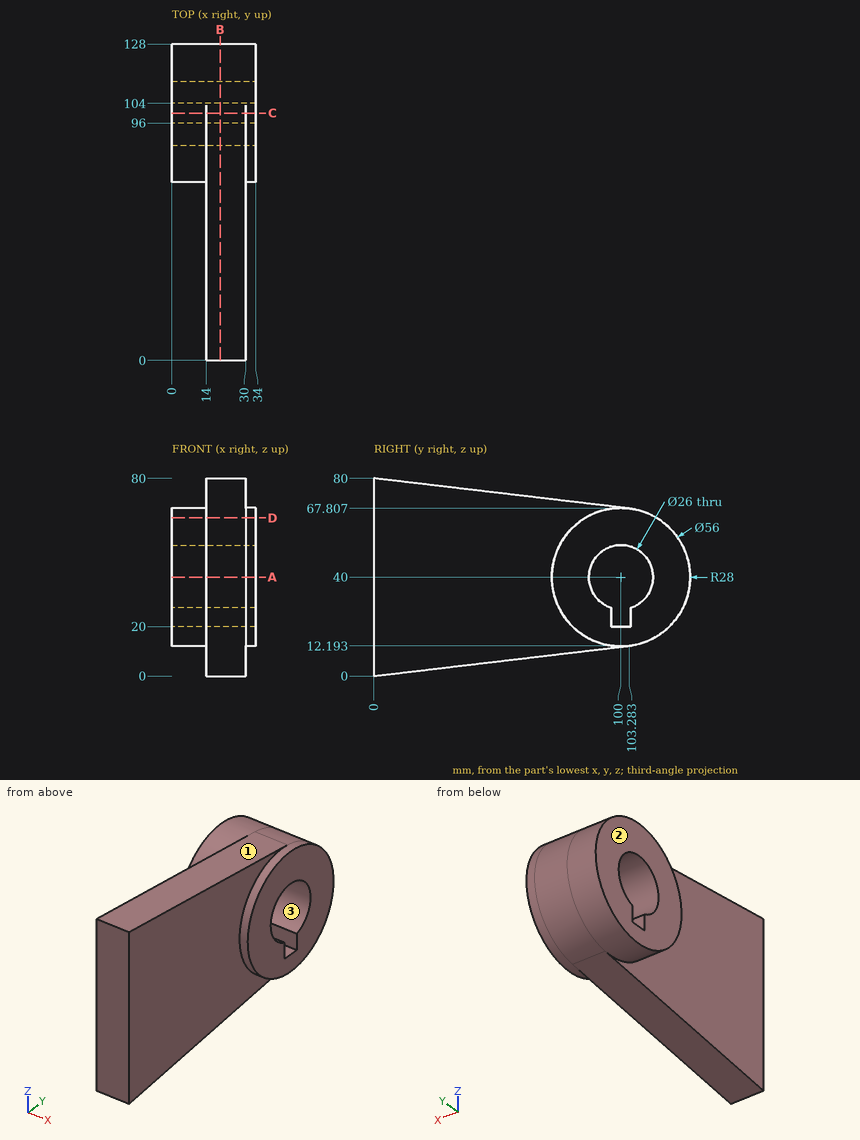
Print and shaded views of the part. All mm, measured from the part's lowest x, y and z. Coordinates: 2 decimals unless noted, no trailing zeros. Write each loop counter-clockwise with the first axis right and the second up, starting at its lowest first coordinate (ties: lowest second). Pieces come first, ordered by that corner, then holes.
(1) Two-plate mould, pull along Y, no slides. Class the marked faces 1, 2 and 3: +Y half, -Y half, draft (parallel to the pull), parting line (faces both ways), or undercut.
(2) Cut at A-A, the plane z = 40. List the corners of the cut face in (x, y).
(3) Cut at D-D, the plane z = 64. List the corners of the cut face in (x, y).
(4) Cut at C-C, the plane y = 100. List the corners of the cut face in (x, z).
(5) Flat gauge pins, fed straight in: pin 1 (2 mm diameter, centred on x = 25.5, y = 85.5, fed in from +Z); pin 2 (4 mm diameter, centred on x = 25.5, y = 52.5, fed in from +Z); pin 3 (5 mm diameter, centred on x = 5, z = 8, fed in from +Y); pin 4 (12 mm diameter, centred on x = 7.5, y = 109, fed in from -Z). Where does each tip first touch, or does it go through?
(6) Drill centre lines: probe 1 along Z at (x, y) = (11, 100); probe 2 along Y at (x, z) = (20, 40); probe 3 along Y at (x, z) = (13, 22). Where is each one in solid material? Low to high.
(7) Cut at B-B, the plane x = 19.5. List the corners of the cut face in (y, z).
Geometry says:
1. face 1: +Y half
1. face 2: draft
1. face 3: undercut
2. outline: (0, 72) - (14, 72) - (14, 0) - (30, 0) - (30, 72) - (34, 72) - (34, 87) - (0, 87) - close; (0, 113) - (34, 113) - (34, 128) - (0, 128) - close
3. outline: (0, 85.58) - (14, 85.58) - (14, 0) - (30, 0) - (30, 85.58) - (34, 85.58) - (34, 114.42) - (0, 114.42) - close
4. outline: (0, 12) - (14, 12) - (14, 11.81) - (30, 11.81) - (30, 12) - (34, 12) - (34, 20) - (0, 20) - close; (0, 53) - (34, 53) - (34, 68) - (30, 68) - (30, 68.19) - (14, 68.19) - (14, 68) - (0, 68) - close
5. pin 1: stops at z = 70.02
5. pin 2: stops at z = 74.04
5. pin 3: passes through
5. pin 4: stops at z = 12.16
6. probe 1: z = 12 to 20, 53 to 68
6. probe 2: y = 0 to 87, 113 to 128
6. probe 3: y = 78.55 to 96, 104 to 121.45
7. outline: (0, 0) - (103.28, 12.19) arc R28 ccw to (103.28, 67.81) - (0, 80) - close; hole (96, 20) - (104, 20) - (104, 27.63) arc R13 ccw (long way) to (96, 27.63) - close
